Can you work these out from the model? Positions are in its coordinate system, mm. Face numbers are marked on the shaded views. A direction names the side the tool comes from. Give positions to 0.01 mm unless a question says otherwise; leave off trailing zeros. Loops run counter-clockwise (first coordinate to the right, second up) from the corner with the lowest first, then second, coordinate; pieces in that order, holes last. Notation, with made-up numbers: M 78,-30.5 L 104,-30.5 A25 cw 104,-10.5 Z; hole C 33,89.5 d8. An arc over 180 degrees is marked long. One line per item, written item: value. Start each with the question number.
from build123d import *

# Parameters (mm, degrees)
F0_R     = 7.8929339783
F1_DEPTH = 9.2
F2_T     = -2.5
F3_DEPTH = 14.5
F4_W     = 39.6901145577
F4_H     = 78.7652172148
F5_DEPTH = 19
F6_R     = 5
F7_T     = -2.5


# Not quite as in the source:
# - a shell that OpenCascade refuses in one call is made with other operations: the cavity is built on its own and cut out


with BuildPart() as f1:
    # F0 (on Front) → F1 (new body)
    with BuildSketch(Plane.XZ):
        Circle(F0_R)
    extrude(amount=F1_DEPTH)

    # F2
    f2_openings = [f1.faces().sort_by_distance(p)[0] for p in [
        (0, -9.2, 0),
    ]]
    offset(amount=F2_T, openings=f2_openings)

    # F3 (add): a face of the model
    f3_faces = [f1.faces().sort_by_distance(p)[0] for p in [
        (0, -2.5, 0),
    ]]
    extrude(f3_faces, amount=F3_DEPTH)

    # F4 (on Front) → F5 (join)
    with BuildSketch(Plane.XZ):
        with Locations((-0.3387015313, 1.4586504549)):
            Rectangle(F4_W, F4_H)
    extrude(amount=-F5_DEPTH)

    # F6
    f6_edges = [f1.edges().sort_by_distance(p)[0] for p in [
        (19.506356, 9.5, 40.841259),
        (19.506356, 9.5, -37.923958),
        (-20.183759, 9.5, 40.841259),
        (-20.183759, 9.5, -37.923958),
    ]]
    fillet(f6_edges, radius=F6_R)

    # F7: a shell. OpenCascade refuses it in one call, so the cavity is built on its own and cut out:
    # the body offset inwards by the wall thickness, plus a prism from it out through each open face.
    f7_core = offset(f1.part, amount=F7_T, kind=Kind.INTERSECTION, mode=Mode.PRIVATE)
    f7_exits = [f7_core.faces().sort_by_distance(p)[0] for p in [
        (17.006356, 9.5, 1.45865),
        (-17.683759, 9.5, 1.45865),
    ]]
    add(f7_core, mode=Mode.SUBTRACT)
    extrude(f7_exits, amount=-F7_T, mode=Mode.SUBTRACT)


solid = f1.part
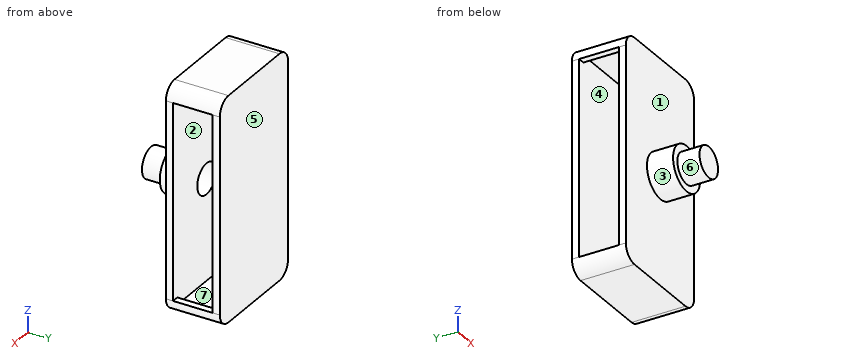
Q1. Which directions (+Z, -Z, +X, -X, +Y, -Y) give clear straight access to the entire face, cutting with the end or side of a thin tool? Please do the marked faces 5, 6 and 7.
Q2. If we section it at C-C, the plane x = -14: Write out the boundary of the cut face in (y, z).
Q3. I need wall thicknesses on line 1 along Y through (x, z) = (-8, -1.5); line 2 along X through (y, z) = (-12, 0); line 3 along X through (y, z) = (0.25, 0). Which ranges of each line are inside material? Lowest first, please.
Q4. For P1, Ø0.8, axis at x = -19.5, y = 6.5, coming from the +Z side; P2, Ø1.2, axis at x = -19, y = 12, coming from the -Z side; P3, Ø8, axis at x = 3, z = 23, coming from the -Y side; P4, Ø6, axis at y = 8, z = -25, coming from the +X side, each with a flat end and sliding along its axis, tell me the tip position at first contact or that it passes through.
Q5. If we section it at B-B, the plane z = 0: Write out the boundary of the cut face in (x, y), plus the area to 3 significant figures.
Q6. If we mould it in two halves opening along Y, with no side actions, what happens to the marked faces 1, 2, 3 and 4? For each: released by +Y, released by -Y, zero draft, split by the parting line, or undercut.
Q7. If we section it at A-A, the plane y = 9: Write out the boundary of the cut face in (x, z), plus the area to 3 significant figures.
Q8. If we section it at D-D, the plane x = 0: Write out the boundary of the cut face in (y, z), plus the area to 3 significant figures.
Response:
1. face 5: +Z, -Z, +X, -X, +Y
1. face 6: -Y
1. face 7: none
2. outline: M 0,-37.92 L 19,-37.92 L 19,40.84 L 0,40.84 Z; hole M 2.5,-35.42 L 16.5,-35.42 L 16.5,38.34 L 2.5,38.34 Z
3. line 1: 0 to 2.5, 16.5 to 19
3. line 2: -5.39 to -2.89, 2.89 to 5.39
3. line 3: -20.18 to -5.39, 5.39 to 19.51
4. P1: z = 38.95
4. P2: z = -36.75
4. P3: y = 0
4. P4: through
5. outline: M -20.18,0 L -7.89,0 L -7.89,-9.2 L -5.39,-9.2 L -5.39,-17 L 5.39,-17 L 5.39,-9.2 L 7.89,-9.2 L 7.89,0 L 19.51,0 L 19.51,2.5 L 5.39,2.5 L 5.39,-6.7 L 2.89,-6.7 L 2.89,-14.5 L -2.89,-14.5 L -2.89,-6.7 L -5.39,-6.7 L -5.39,2.5 L -20.18,2.5 Z; M -20.18,16.5 L 19.51,16.5 L 19.51,19 L -20.18,19 Z
5. area: 283 mm^2
6. face 1: released by -Y
6. face 2: undercut
6. face 3: zero draft
6. face 4: undercut
7. outline: M -20.18,-32.92 A5 ccw -15.18,-37.92 L 14.51,-37.92 A5 ccw 19.51,-32.92 L 17.01,-32.92 A2.5 cw 14.51,-35.42 L -15.18,-35.42 A2.5 cw -17.68,-32.92 Z; M -20.18,35.84 L -17.68,35.84 A2.5 cw -15.18,38.34 L 14.51,38.34 A2.5 cw 17.01,35.84 L 19.51,35.84 A5 ccw 14.51,40.84 L -15.18,40.84 A5 ccw Z
7. area: 207 mm^2
8. outline: M -17,-5.39 L -9.2,-5.39 L -9.2,-7.89 L 0,-7.89 L 0,-37.92 L 19,-37.92 L 19,40.84 L 0,40.84 L 0,7.89 L -9.2,7.89 L -9.2,5.39 L -17,5.39 Z; hole M -14.5,-2.89 L -6.7,-2.89 L -6.7,-5.39 L 2.5,-5.39 L 2.5,-35.42 L 16.5,-35.42 L 16.5,38.34 L 2.5,38.34 L 2.5,5.39 L -6.7,5.39 L -6.7,2.89 L -14.5,2.89 Z
8. area: 549 mm^2
